Here's the drawing with two shaded views (mm, measured from the low corner). I have some questions. A direction names the side the tool comes from. Round coordinates to 2 decimals unless told otherwise and drop trailing zeros. Loops run counter-clockwise (first coordinate to the right, second up) from the corner with the lowest first, then second, coordinate; pieces in that order, holes last.
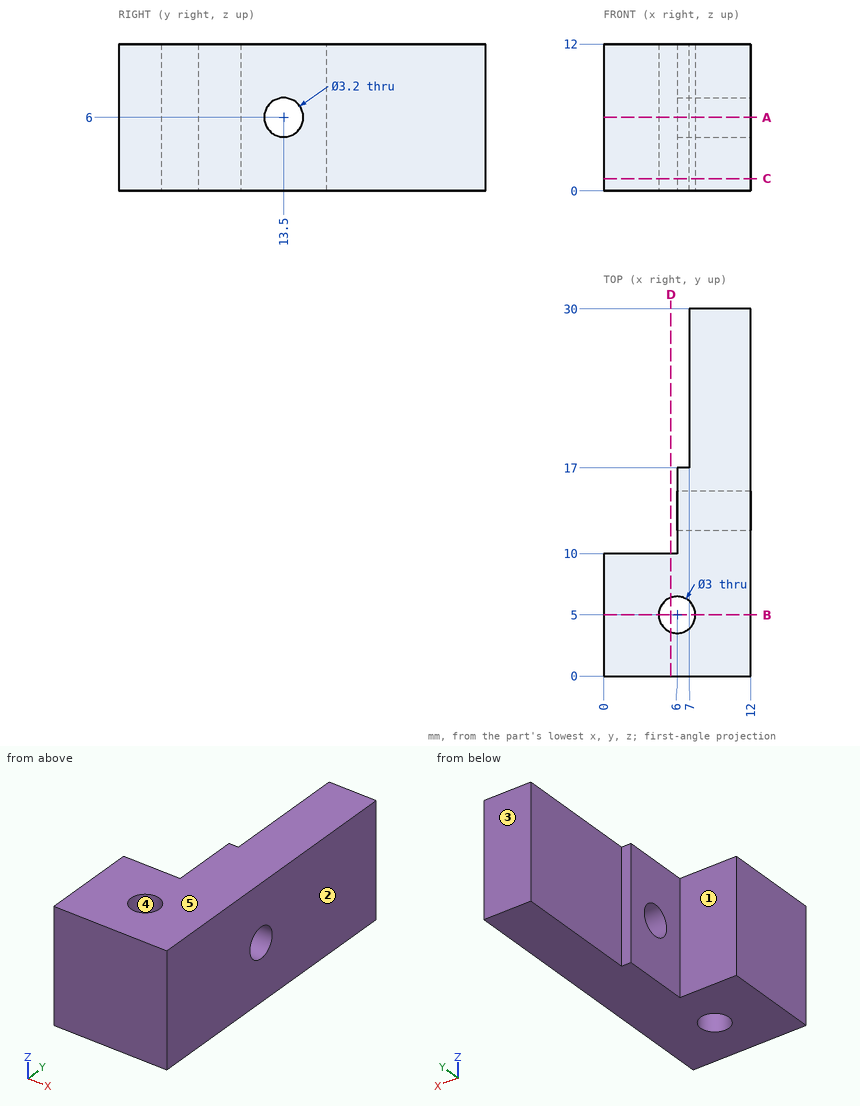
(1) For the marked faces 1 and 2, which set-ups out of +Z, -Z, +X, -X, +Y, -Y let a thin tool reach every point of the face, with its end or its side?
Worked answers:
face 1: +Z, -Z, -X, +Y
face 2: +Z, -Z, +X, +Y, -Y
(2) If we section it at A-A, the plane z = 6: List the corners of the cut face in (x, y) for me, then the cut area to 3 significant figures.
Worked answers:
outline: (0, 0) - (12, 0) - (12, 11.9) - (6, 11.9) - (6, 10) - (0, 10) - close; (6, 15.1) - (12, 15.1) - (12, 30) - (7, 30) - (7, 17) - (6, 17) - close; hole circle Ø3 at (6, 5)
area: 201 mm2
(3) Will these pins go through, and if not, where does the flat tip stop? P1, Ø3, axis at x = 3.5, z = 4, coming from the +Y side; P2, Ø5, axis at y = 13.5, z = 6, coming from the -X side.
Worked answers:
P1: stops at y = 10
P2: stops at x = 6
(4) If we section it at D-D, the plane x = 5.5: List the corners of the cut face in (y, z) for me.
Worked answers:
outline: (0, 0) - (3.59, 0) - (3.59, 12) - (0, 12) - close; (6.41, 0) - (10, 0) - (10, 12) - (6.41, 12) - close
(5) If I drill on line 1 (Z direction, x = 8.55, y = 13.5); line 2 (X direction, y = 10.75, z = 3.75); line 3 (X direction, y = 18, z = 5.25), over which ranges is the centre line in solid material (lowest first)?
Worked answers:
line 1: z = 0 to 4.4, 7.6 to 12
line 2: x = 6 to 12
line 3: x = 7 to 12
(6) If we section it at B-B, the plane y = 5: List the corners of the cut face in (x, z) for me.
Worked answers:
outline: (0, 0) - (4.5, 0) - (4.5, 12) - (0, 12) - close; (7.5, 0) - (12, 0) - (12, 12) - (7.5, 12) - close
(7) If we mould it in two halves opening along Y, with no side actions, what happens to the marked faces 3, 4 and 5? For each: released by +Y, released by -Y, zero draft, split by the parting line, or undercut.
Worked answers:
face 3: released by +Y
face 4: undercut
face 5: zero draft
(8) If we section it at C-C, the plane z = 1: List the corners of the cut face in (x, y) for me, then the cut area to 3 significant figures.
Worked answers:
outline: (0, 0) - (12, 0) - (12, 30) - (7, 30) - (7, 17) - (6, 17) - (6, 10) - (0, 10) - close; hole circle Ø3 at (6, 5)
area: 220 mm2
